Design review of the part built by this model. Coordinates are the model's own, in mm. Face numbers are marked on the shaded views. A direction names the side the tool comes from. Coordinates: 2 decimals unless noted, no trailing zeros. Loops run counter-clockwise (first coordinate to the right, second up) from the corner with the lowest first, then second, coordinate; pieces in that order, holes last. Notation, with made-up numbers: M 75.25,-23.5 L 126.25,-23.5 A20 cw 126.25,13.5 Z; hole C 42.5,47.25 d8. An arc over 180 degrees is marked long. Answer as CSV lines item,"result". Start each with the question number.
from build123d import *

# Parameters (mm, degrees)
BOSS_EXTRUDE1_DEPTH = 38.1
SKETCH2_R           = 3.175
CUT_EXTRUDE1_DEPTH  = 39.1


with BuildPart() as part:
    # Sketch1 → Boss-Extrude1 (new body)
    with BuildSketch(Plane(origin=(0, 0, 0), x_dir=(1, 0, 0), z_dir=(0, 1, 0))):
        with BuildLine():
            Line((1.047492977, 4.970830762), (0.644904142, 6.175331583))
            Line((0.644904142, 6.175331583), (-0.556834652, 6.175331583))
            Line((-0.556834652, 6.175331583), (-0.991979734, 4.982205958))
            ThreePointArc((-0.991979734, 4.982205958), (-1.917824995, 4.70407773), (-2.774218752, 4.255597527))
            Line((-2.774218752, 4.255597527), (-3.910602747, 4.822634931))
            Line((-3.910602747, 4.822634931), (-4.760360397, 3.97287728))
            Line((-4.760360397, 3.97287728), (-4.224387215, 2.821516022))
            ThreePointArc((-4.224387215, 2.821516022), (-4.682392321, 1.970178203), (-4.970830762, 1.047492977))
            Line((-4.970830762, 1.047492977), (-6.175331583, 0.644904142))
            Line((-6.175331583, 0.644904142), (-6.175331583, -0.556834652))
            Line((-6.175331583, -0.556834652), (-4.982205958, -0.991979734))
            ThreePointArc((-4.982205958, -0.991979734), (-4.70407773, -1.917824995), (-4.255597527, -2.774218752))
            Line((-4.255597527, -2.774218752), (-4.822634931, -3.910602747))
            Line((-4.822634931, -3.910602747), (-3.97287728, -4.760360397))
            Line((-3.97287728, -4.760360397), (-2.821516022, -4.224387215))
            ThreePointArc((-2.821516022, -4.224387215), (-1.970178203, -4.682392321), (-1.047492977, -4.970830762))
            Line((-1.047492977, -4.970830762), (-0.644904142, -6.175331583))
            Line((-0.644904142, -6.175331583), (0.556834652, -6.175331583))
            Line((0.556834652, -6.175331583), (0.991979734, -4.982205958))
            ThreePointArc((0.991979734, -4.982205958), (1.917824995, -4.70407773), (2.774218752, -4.255597527))
            Line((2.774218752, -4.255597527), (3.910602747, -4.822634931))
            Line((3.910602747, -4.822634931), (4.760360397, -3.97287728))
            Line((4.760360397, -3.97287728), (4.224387215, -2.821516022))
            ThreePointArc((4.224387215, -2.821516022), (4.682392321, -1.970178203), (4.970830762, -1.047492977))
            Line((4.970830762, -1.047492977), (6.175331583, -0.644904142))
            Line((6.175331583, -0.644904142), (6.175331583, 0.556834652))
            Line((6.175331583, 0.556834652), (4.982205958, 0.991979734))
            ThreePointArc((4.982205958, 0.991979734), (4.70407773, 1.917824995), (4.255597527, 2.774218752))
            Line((4.255597527, 2.774218752), (4.822634931, 3.910602747))
            Line((4.822634931, 3.910602747), (3.97287728, 4.760360397))
            Line((3.97287728, 4.760360397), (2.821516022, 4.224387215))
            ThreePointArc((2.821516022, 4.224387215), (1.970178203, 4.682392321), (1.047492977, 4.970830762))
        make_face()
    extrude(amount=BOSS_EXTRUDE1_DEPTH)

    # Sketch2 → Cut-Extrude1 (cut, through all)
    with BuildSketch(Plane(origin=(0, 38.1, 0), x_dir=(1, 0, 0), z_dir=(0, 1, 0))):
        Circle(SKETCH2_R)
    extrude(amount=-CUT_EXTRUDE1_DEPTH, mode=Mode.SUBTRACT)


solid = part.part
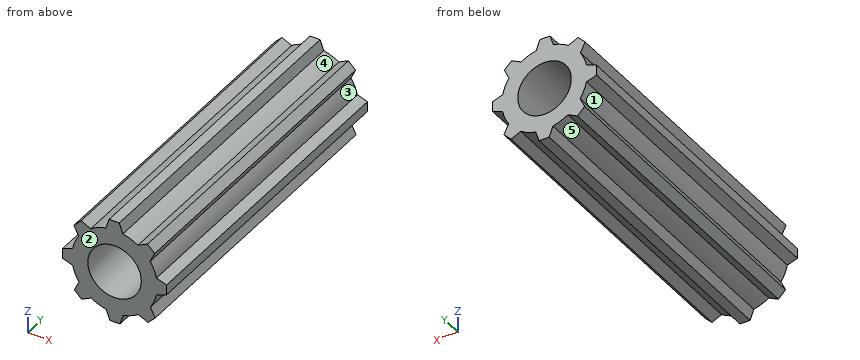
Item 1: For line 1 along Z through (x, y) = (0, 9.5) (3 decimals); line 2 along X through (y, z) = (14, -2.5), list the stretches that pass through material, from the lowest coordinate up. Write a range as from..to.
Item 2: For pin 1 (2 mm diameter, centred on y = 5, z = -4.5, fed in from -X); pin 2 (1.5 mm diameter, centred on x = -1, z = 0.5, fed in from -Y), all flat-tipped, find the tip position at first contact; note any pin that passes through.
Item 3: Add section A-A (x = 0). Give the boundary of the cut face in (y, z) (3 decimals), plus the area to 3 significant figures.
Item 4: Mouldability with a two-part tool opening along Z and no side actions: class the marked faces 3, 4 and 5 as released by +Z, released by -Z, zero draft, split by the parting line, or undercut.
Item 5: For the marked faces 1 and 2, list the 3-axis set-ups (+Z, -Z, +X, -X, +Y, -Y) from which the entire face can be reached by the end or side of a thin tool; tool diameter is ignored.
Item 6: Add section B-B (z = 0). Give the boundary of the cut face in (x, y) (3 decimals).
Response:
1,line 1,"-6.175..-3.175, 3.175..6.175"
1,line 2,"-4.42..-1.96, 1.96..4.42"
2,pin 1,"x = -4.76"
2,pin 2,"through"
3,outline,"M 0,-6.175 L 38.1,-6.175 L 38.1,-3.175 L 0,-3.175 Z; M 0,3.175 L 38.1,3.175 L 38.1,6.175 L 0,6.175 Z"
3,area,"229 mm²"
4,face 3,"undercut"
4,face 4,"released by +Z"
4,face 5,"released by -Z"
5,face 1,"-X, +Y, -Y"
5,face 2,"+Z, -Z, +X, -X, -Y"
6,outline,"M -6.175,0 L -3.175,0 L -3.175,38.1 L -6.175,38.1 Z; M 3.175,0 L 6.175,0 L 6.175,38.1 L 3.175,38.1 Z"
